Job drawing, mm, ordinate dimensions from the low corner. One solid piece. A direction names the side the tool comes from. Round coordinates to 2 decimals unless told otherwise and drop trailing zeros. Order: outer loops, then holes, each group sorted by start corner. A loop starts at its lowest first (then second) coordinate and runs counter-clockwise, first axis right, second up. Notation, with made-up numbers: (22, 70) -> (63, 70) arc R22 ccw to (63, 94) -> close; hole circle Ø6 at (48.25, 54). An arc over 180 degrees is marked (long way). Return JSON: item names as keys, results as strings. Group by question number.
Q1. Mould opens along Z. For the marked faces 4, 5 and 6 say: +Z half, -Z half, draft (parallel to the pull), parting line (faces both ways), or undercut.
Q2. Flat gauge pins, fed straight in: pin 1 (3 mm diameter, centred on x = 20, y = 13, fed in from +Z); pin 2 (12 mm diameter, centred on x = 35.5, y = 9.5, fed in from +Z); pin 3 (6 mm diameter, centred on x = 6.5, y = 17.5, fed in from -Z). Where does each tip first touch, or does it go through?
Q3. Cut at A-A (y = 15.75). Write the cut outline in (x, z).
Q4. Probe line 1 along Y through (x, z) = (37, 33); line 2 along Z through (x, y) = (28.5, 16.75) (1 decimal); line 3 along Z through (x, y) = (12, 15.5). List the from-to ranges inside material, lowest first.
Q5. Which spindle directions (+Z, -Z, +X, -X, +Y, -Y) get a long thin tool onto all of the face, cutting with end or side? Do the marked faces 1, 2 and 3. Say none if no direction does.
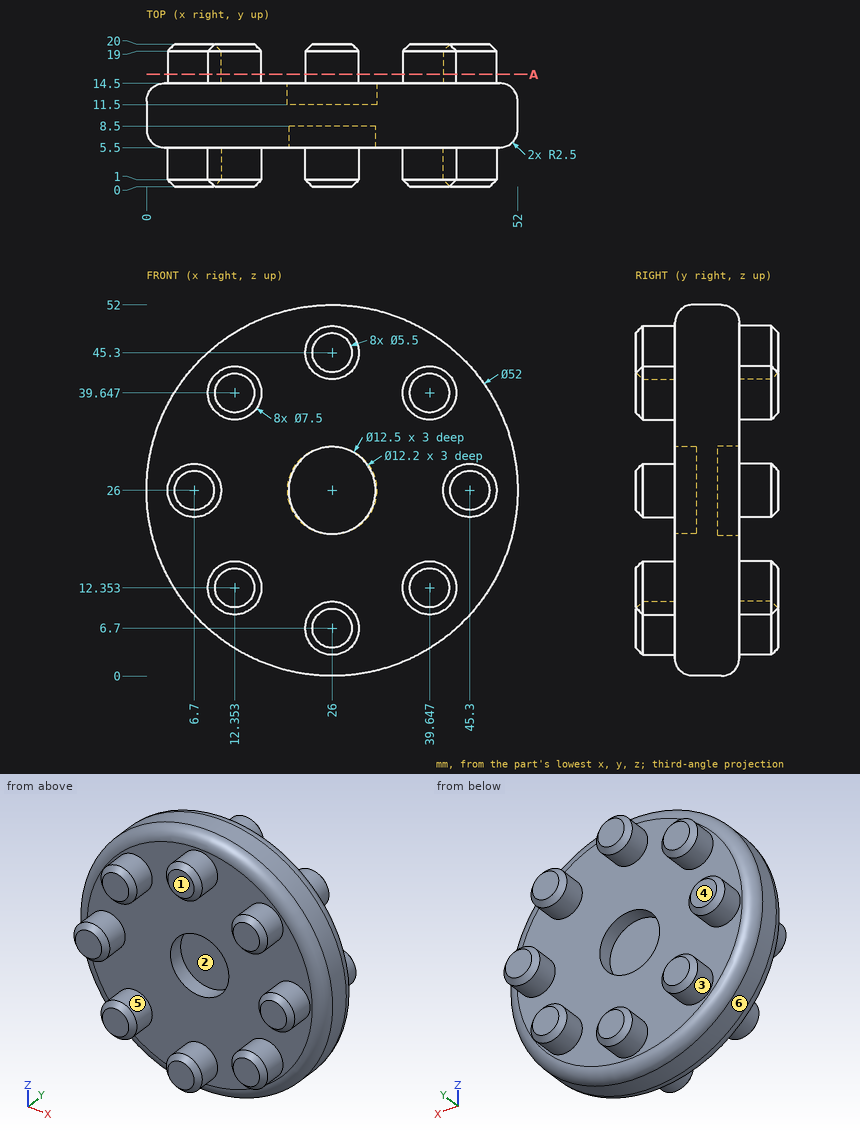
Solution:
{
 "1": {"face 4": "draft", "face 5": "undercut", "face 6": "parting line"},
 "2": {"pin 1": "stops at z = 51.56", "pin 2": "stops at z = 51.76", "pin 3": "stops at z = 9.92"},
 "3": {"outline": "circle Ø7.5 at (6.7, 26); circle Ø7.5 at (12.35, 12.35); circle Ø7.5 at (12.35, 39.65); circle Ø7.5 at (26, 6.7); circle Ø7.5 at (26, 45.3); circle Ø7.5 at (39.65, 12.35); circle Ø7.5 at (39.65, 39.65); circle Ø7.5 at (45.3, 26)"},
 "4": {"line 1": "y = 5.5 to 14.5", "line 2": "z = 3.9 to 9.5, 42.5 to 48.1", "line 3": "z = 8.62 to 16.09, 35.91 to 43.38"},
 "5": {"face 1": "+Z, -Z, +X, -X, -Y", "face 2": "-Y", "face 3": "+Y"}
}
